Input: part model. Units: mm. Frame: model coordinates. Face numbers are marked on the shaded views. A direction names the side the tool comes from. Coordinates: 2 decimals unless noted, no trailing zeros. Loops run counter-clockwise (first coordinate to the right, second up) from the corner with the lowest first, then second, coordinate; pieces in that order, holes last. Notation, with made-up numbers: (13.25, -37) -> (61.25, -37) arc R19 cw to (61.25, -28) -> close; hole circle Ø2 at (60, 23). An arc over 180 degrees is marked (long way). Answer as a JSON object with one key per item and string values.
from build123d import *

# Parameters (mm, degrees)
F0_W      = 63.5
F0_H      = 25.4
F1_DEPTH  = 12.7
F2_R      = 12.5320537087
F3_DEPTH  = 12.7
F5_DEPTH  = 12.7
F6_W      = 31.5867842689
F6_H      = 25.4
F7_DEPTH  = 12.7
F8_R      = 15.875
F9_DEPTH  = 25.4
F10_R     = 6.985
F11_DEPTH = 25.4


with BuildPart() as f1:
    # F0 (on Top) → F1 (new body)
    with BuildSketch(Plane.XY):
        with Locations((31.75, 12.7)):
            Rectangle(F0_W, F0_H)
    extrude(amount=F1_DEPTH)

    # F2 (on face) → F3 (join)
    with BuildSketch(Plane.XY.offset(12.7)):
        with Locations((63.5, 12.7)):
            Circle(F2_R)
    extrude(amount=-F3_DEPTH)

    # F4 (on face) → F5 (cut)
    with BuildSketch(Plane.XY.offset(12.7)):
        with BuildLine():
            ThreePointArc((63.5, 6.0999503105), (67.882802657, 8.0165452354), (69.6845581875, 12.4477947483))
            ThreePointArc((69.6845581875, 12.4477947483), (67.824686248, 16.9379228088), (63.3345581875, 18.7977947483))
            Line((63.3345581875, 18.7977947483), (63.5, 6.0999503105))
        make_face()
        with BuildLine():
            Line((63.5, 6.0999503105), (63.3345581875, 18.7977947483))
            ThreePointArc((63.3345581875, 18.7977947483), (56.9867066583, 12.6129642476), (63.0043309564, 6.1063871778))
            Line((63.0043309564, 6.1063871778), (63.5, 6.0999503105))
        make_face()
        with BuildLine():
            ThreePointArc((63.0043309564, 6.1063871778), (56.9867066583, 12.6129642476), (63.3345581875, 18.7977947483))
            Line((63.3345581875, 18.7977947483), (44.4543498473, 19.0477740161))
            ThreePointArc((44.4543498473, 19.0477740161), (48.8354076377, 17.1302891933), (50.6362277486, 12.7))
            ThreePointArc((50.6362277486, 12.7), (48.7763558091, 8.2098719395), (44.2862277486, 6.35))
            Line((44.2862277486, 6.35), (44.2862277486, 6.3494645845))
            Line((44.2862277486, 6.3494645845), (63.0043309564, 6.1063871778))
        make_face()
        with BuildLine():
            ThreePointArc((63.0043309564, 6.1063871778), (63.2521026428, 6.0983301187), (63.5, 6.0999503105))
            Line((63.5, 6.0999503105), (63.0043309564, 6.1063871778))
        make_face()
        with BuildLine():
            Line((44.2862277486, 19.05), (44.4543498473, 19.0477740161))
            ThreePointArc((44.4543498473, 19.0477740161), (44.3702961658, 19.0494434796), (44.2862277486, 19.05))
        make_face()
        with BuildLine():
            ThreePointArc((50.6362277486, 12.7), (48.8354076377, 17.1302891933), (44.4543498473, 19.0477740161))
            Line((44.4543498473, 19.0477740161), (44.2862277486, 19.05))
            Line((44.2862277486, 19.05), (44.2862277486, 6.35))
            ThreePointArc((44.2862277486, 6.35), (48.7763558091, 8.2098719395), (50.6362277486, 12.7))
        make_face()
        with BuildLine():
            Line((44.2862277486, 6.35), (44.2862277486, 19.05))
            ThreePointArc((44.2862277486, 19.05), (37.9362277486, 12.7), (44.2862277486, 6.35))
        make_face()
    extrude(amount=-F5_DEPTH, mode=Mode.SUBTRACT)

    # F6 (on face) → F7 (join)
    with BuildSketch(Plane.XY.offset(12.7)):
        with Locations((15.7933921345, 12.7)):
            Rectangle(F6_W, F6_H)
    extrude(amount=F7_DEPTH)

    # F8 (on face) → F9 (join)
    with BuildSketch(Plane.XZ):
        with Locations((15.7933921345, 25.4)):
            Circle(F8_R)
    extrude(amount=-F9_DEPTH)

    # F10 (on face) → F11 (cut)
    with BuildSketch(Plane.XZ):
        with Locations((15.7933921345, 28.575)):
            Circle(F10_R)
    extrude(amount=-F11_DEPTH, mode=Mode.SUBTRACT)


solid = f1.part
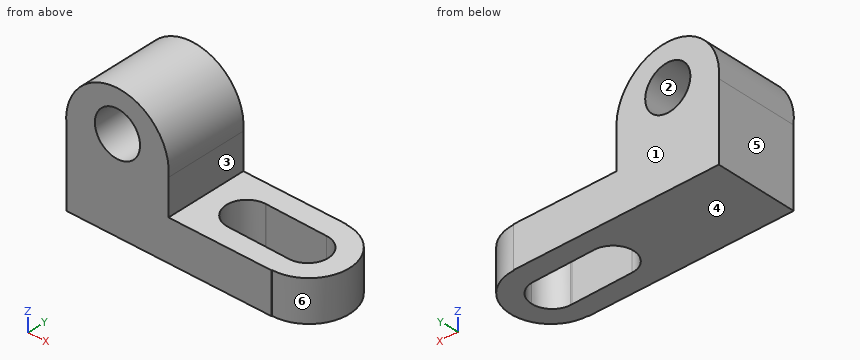
1. Access query for the marked faces 5 and 6. Directions: +Z, -Z, +X, -X, +Y, -Y. A direction counts if a zero-diameter tool reaches every point of the face in a straight line with its end or side. Return the directions, or none.
Reply:
{"face 5": "-Z, -X, +Y, -Y", "face 6": "+Z, -Z, +X"}
2. Section query C-C (y = 9.75). Return loops of the section in (x, z) (3 decimals), plus the area to 3 significant figures.
Reply:
{"outline": "(0, 0) -> (38.663, 0) -> (38.663, 12.7) -> (31.587, 12.7) -> (31.587, 23.792) arc R15.875 ccw (long way) to (0, 23.792) -> close; (69.083, 0) -> (75.68, 0) -> (75.68, 12.7) -> (69.083, 12.7) -> close; hole circle Ø13.97 at (15.793, 28.575)", "area": "1,220 mm2"}
3. Section query D-D (y = 22). Return loops of the section in (x, z) (3 decimals), plus the area to 3 significant figures.
Reply:
{"outline": "(0, 0) -> (71.9, 0) -> (71.9, 12.7) -> (31.587, 12.7) -> (31.587, 23.792) arc R15.875 ccw (long way) to (0, 23.792) -> close; hole circle Ø13.97 at (15.793, 28.575)", "area": "1,560 mm2"}
4. Pin query (flat end, axial travel): P1, Ø7, axis at y = 17.5, z = 8, coming from the -X side; P2, Ø5.5, axis at y = 11, z = 16.5, coming from the +X side; P3, Ø1, axis at y = 10, z = 36.5, coming from the +X side. Return the tip coordinate at first contact, or that it passes through.
Reply:
{"P1": "stops at x = 0", "P2": "stops at x = 31.59", "P3": "stops at x = 27.61"}
5. Section query A-A (x = 52). Return loops of the section in (y, z), plus the area to 3 significant figures.
Reply:
{"outline": "(0, 0) -> (6.25, 0) -> (6.25, 12.7) -> (0, 12.7) -> close; (18.95, 0) -> (25.4, 0) -> (25.4, 12.7) -> (18.95, 12.7) -> close", "area": "161 mm2"}
6. Mould query, pull axis Z, two halves, no side actions, for the marked faces 1, 2, 3 and 4. Classes: pulls with the +Z half, pulls with the -Z half, needs draft (parallel to the pull), parting line crosses it, or undercut.
Reply:
{"face 1": "needs draft", "face 2": "undercut", "face 3": "undercut", "face 4": "pulls with the -Z half"}
7. Line query: line 1 along X through (y, z) = (3, 18); line 2 along Z through (x, y) = (19, 14.75); line 3 along Z through (x, y) = (10.5, 17.5). Output: solid intervals per line, ascending.
Reply:
{"line 1": "x = 0 to 31.59", "line 2": "z = 0 to 22.37, 34.78 to 40.95", "line 3": "z = 0 to 24.02, 33.13 to 40.37"}
